Read the model definition and answer for the solid it produces. Units are mm, in the model's axes. A direction names the side the tool comes from. Give positions to 0.01 mm unless a question says otherwise; leave off trailing zeros. Write each loop counter-clockwise with the first axis right and the second up, starting at its lowest first coordinate (ties: lowest second). Pieces come first, ordered by that corner, then holes. Notation, with made-up numbers: M 50.5,57.5 L 70.5,57.5 A27 cw 70.5,86.5 Z; hole C 23,27.5 d1. An arc over 180 degrees is marked long. Use a Markdown table: item, result. Add a question column.
Item 1: A cutting plane is placed at A-A on z = -9.5. Determine the outline of the cut face in (x, y).
Item 2: For faces 1 (the flat face through (10, 12.5, 11)), 2 (the flat face through (0.5, 10.5, -11)), 3 (the cylindrical face through (7.55, -5.26, 2.52)), determine the directions among +Z, -Z, +X, -X, +Y, -Y from which every point of the face is accessible in a straight line to the end or side of a thin tool.
Item 3: The mould has two halves that part along Z. Classify faces 4 (the flat face through (0.5, 10.5, 11)), 5 (the flat face through (10, 14.5, -11)), 6 (the flat face through (10, 0, -10)): pulls with the +Z half, pulls with the -Z half, needs draft (parallel to the pull), parting line crosses it, or undercut.
Item 4: Given P1, Ø3, axis at y = -6, z = 5, coming from the +X side; P2, Ø5, axis at x = 8, z = 0.5, coming from the +Y side; P3, Ø3.5, axis at x = 14.5, y = 4.5, coming from the -Z side, each flat-ended and moving along its own axis, determine where each tip first touches the part or whether it passes through.
Item 5: Consider probe 1 along Y at (x, z) = (3.5, -0.5); probe 2 along Z at (x, y) = (18.5, 12.25); probe 3 along Z at (x, y) = (18, 3.5). Determine where each line is inside the solid, lowest interval first. Write a range as [from, to].
Item 6: A cutting plane is placed at B-B on y = 3.5. Determine the outline of the cut face in (x, z).
Item 7: A cutting plane is placed at D-D on y = -4.75. Determine the outline of the cut face in (x, z), then the cut area to 3 significant figures.
Autodesk Inventor part; units mm, degrees
ref_plane "YZ Plane" through (0, 0, 0) normal (1, 0, 0) x (0, 1, 0)
ref_plane "XZ Plane" through (0, 0, 0) normal (0, 1, 0) x (-1, 0, 0)
ref_plane "XY Plane" through (0, 0, 0) normal (0, 0, 1) x (1, 0, 0)
sketch "Sketch1" plane through (0, 0, 0) normal (1, 0, 0) x (0, 1, 0)
  line L0 (0, 8) -> (0, -8)
  line L1 (0, -8) -> (11, -8)
  line L2 (0, 8) -> (11, 8)
  line L3 (11, 8) -> (11, 13)
  line L4 (11, 13) -> (12.5, 13)
  line L5 (12.5, 13) -> (12.5, 8)
  line L6 (12.5, 8) -> (14.5, 8)
  line L7 (14.5, 8) -> (14.5, 15)
  line L8 (14.5, 15) -> (9, 15)
  line L9 (9, 15) -> (9, 10)
  line L10 (9, 10) -> (-3, 10)
  line L11 (-3, 10) -> (-4, 10)
  line L12 (-4, 10) -> (-4, 2.5)
  line L13 (0, 0) -> (3.5, 0)
  line L14 (0, -8) -> (11, -8)
  line L15 (11, -8) -> (11, -13)
  line L16 (11, -13) -> (12.5, -13)
  line L17 (12.5, -13) -> (12.5, -8)
  line L18 (14.5, -8) -> (14.5, -15)
  line L19 (14.5, -15) -> (9, -15)
  line L20 (9, -15) -> (9, -10)
  line L21 (9, -10) -> (-3, -10)
  line L22 (-3, -10) -> (-4, -10)
  line L23 (-4, -10) -> (-4, 2.5)
  line L24 (14.5, -8) -> (12.5, -8)
  point P0 (11.75, -15)
  point P1 (11.75, -13)
  dimension "d0" = 16
  dimension "d1" = 0
  dimension "d2" = 11
  dimension "d3" = 11
  dimension "d4" = 5
  dimension "d5" = 1.5
  dimension "d6" = 2
  dimension "d7" = 7
  dimension "d8" = 5.5
  dimension "d9" = 5
  dimension "d10" = 1
  dimension "d13" = 2
  dimension "d14" = 4
extrude "Extrusion1" add sketch "Sketch1" along normal blind 20
fillet "Fillet1" radius 5 2 edges at (10, 9, -10) (10, 9, 10)
chamfer "Chamfer1" distance 1 angle 45 12 edges at (20, 11, -10.5) (20, 11.75, -13) (20, 12.5, -10.5) (20, 11, 10.5) (20, 11.75, 13) (20, 12.5, 10.5) (0, 11, -10.5) (0, 11.75, -13) (0, 12.5, -10.5) (0, 11, 10.5) (0, 11.75, 13) (0, 12.5, 10.5)
sketch "Sketch3" plane through (0, -4, -10) normal (0, -1, 0) x (1, 0, 0)
  line L0 (13.95, 6.05) -> (6.05, 6.05)
  line L1 (6.05, 6.05) -> (6.05, 13.95)
  line L2 (6.05, 13.95) -> (13.95, 13.95)
  line L3 (13.95, 13.95) -> (13.95, 6.05)
  line L4 (20, 20) -> (20, 0)
  line L5 (0, -5) -> (20, -5)
  point P0 (0, 10)
  point P1 (20, 10)
  dimension "d28" = 7.9
  dimension "d29" = 7.9
  dimension "d30" = 6.05
  dimension "d31" = 11.05
extrude "Extrusion3" add sketch "Sketch3" along normal blind 2.49
sketch "Sketch4" plane through (0, -6.49, -10) normal (0, -1, 0) x (1, 0, 0)
  line L0 (18.45, 6.05) -> (1.55, 6.05)
  line L1 (1.55, 6.05) -> (1.55, 13.95)
  line L2 (1.55, 13.95) -> (18.45, 13.95)
  line L3 (18.45, 13.95) -> (18.45, 6.05)
  line L4 (6.05, 6.05) -> (13.95, 6.05)
  line L5 (13.95, 13.95) -> (6.05, 13.95)
  line L6 (20, 20) -> (20, 0)
  point P0 (0, 10)
  point P1 (18.45, 10)
  dimension "d34" = 0
  dimension "d35" = 0
  dimension "d36" = 16.9
  dimension "d37" = 1.55
extrude "Extrusion4" add sketch "Sketch4" along normal blind 3
fillet "Fillet2" radius 5 4 edges at (18.45, -7.99, -3.95) (13.95, -5.245, -3.95) (6.05, -5.245, 3.95) (1.55, -7.99, 3.95)
sketch "Sketch2" plane through (0, 0, 8) normal (0, 1, 0) x (1, 0, 0)
  circle A0 centre (10, 7.5) radius 3
  line L0 (20, 16) -> (20, 0)
  line L1 (0, -7) -> (20, -7)
  line L2 (0, 0) -> (20, 0)
  point P0 (0, 8)
  dimension "d19" = 6
  dimension "d20" = 10
  dimension "d27" = 7.5
properties part number "Drziak_4"
Filled in:
| question | item | result |
|---|---|---|
| 1 | outline | M 0,-4 L 20,-4 L 20,10 L 19,11 L 1,11 L 0,10 Z; M 0,13.5 L 1,12.5 L 19,12.5 L 20,13.5 L 20,14.5 L 0,14.5 Z |
| 2 | face 1 | +X, -X |
| 2 | face 2 | -X |
| 2 | face 3 | +Z, -X |
| 3 | face 4 | undercut |
| 3 | face 5 | needs draft |
| 3 | face 6 | pulls with the -Z half |
| 4 | P1 | x = 18.45 |
| 4 | P2 | y = 0 |
| 4 | P3 | z = -10.53 |
| 5 | probe 1 | [-9.49, -6.49], [-4, 0] |
| 5 | probe 2 | [-15, -13], [13, 15] |
| 5 | probe 3 | [-10, -8], [8, 10] |
| 6 | outline | M 0,-10 L 20,-10 L 20,-8 L 0,-8 Z; M 0,8 L 20,8 L 20,10 L 0,10 Z |
| 7 | outline | M 6.05,-3.95 L 13.45,-3.95 A5 ccw 13.95,-3.92 L 13.95,3.95 L 11.05,3.95 A5 ccw 6.05,-1.05 Z |
| 7 | area | 57.0 mm² |
